```python
from build123d import *

# Parameters (mm, degrees)
EXTRUDE_1_DEPTH     = 5
FILLET_1_R          = 3
SKETCH_11_R         = 2
CUT_EXTRUDE_6_DEPTH = 88.5
SKETCH_12_R         = 2
CUT_EXTRUDE_7_DEPTH = 88.5


with BuildPart() as part:
    # 스케치1 → 보스-돌출1 (new body)
    with BuildSketch(Plane(origin=(0, 0, 0), x_dir=(1, 0, 0), z_dir=(0, 1, 0))):
        Polygon((-60, -30), (-30, -60), (-12.5, -60), (-12.5, -75), (12.5, -75), (12.5, -60), (30, -60), (60, -30), (60, -12.5), (75, -12.5), (75, 12.5), (60, 12.5), (60, 30), (30, 60), (12.5, 60), (12.5, 75), (-12.5, 75), (-12.5, 60), (-30, 60), (-60, 30), (-60, 12.5), (-75, 12.5), (-75, -12.5), (-60, -12.5), align=None)
    extrude(amount=EXTRUDE_1_DEPTH)

    # 필렛1
    fillet_1_edges = [part.edges().sort_by_distance(p)[0] for p in [
        (-12.5, 2.5, -75),
        (12.5, 2.5, -75),
        (75, 2.5, -12.5),
        (75, 2.5, 12.5),
        (12.5, 2.5, 75),
        (-12.5, 2.5, 75),
        (-75, 2.5, 12.5),
        (-75, 2.5, -12.5),
    ]]
    fillet(fillet_1_edges, radius=FILLET_1_R)

    # 스케치11 → 컷-돌출6 (cut, through all)
    with BuildSketch(Plane.XY.offset(12.5)):
        with Locations((-70, 2.5)):
            Circle(SKETCH_11_R)
        with Locations((70, 2.5)):
            Circle(SKETCH_11_R)
    extrude(amount=-CUT_EXTRUDE_6_DEPTH, mode=Mode.SUBTRACT)

    # 스케치12 → 컷-돌출7 (cut, through all)
    with BuildSketch(Plane.ZY.offset(12.5)):
        with Locations((-70, 2.5)):
            Circle(SKETCH_12_R)
        with Locations((70, 2.5)):
            Circle(SKETCH_12_R)
    extrude(amount=-CUT_EXTRUDE_7_DEPTH, mode=Mode.SUBTRACT)


solid = part.part
```
Geometry check sheet. Reference: the model listing, model coordinates, mm. A direction names the side the tool comes from. Coordinates: 2 decimals unless noted, no trailing zeros. Loops run counter-clockwise (first coordinate to the right, second up) from the corner with the lowest first, then second, coordinate; pieces in that order, holes last.
Item 1: Sectioned sample at D-D, the plane x = 50.5. Record the boundary of the cut face in (y, z), then the cut area to 3 significant figures.
Item 2: Sectioned sample at C-C, the plane z = 36.5. Record the boundary of the cut face in (x, y).
Item 3: Go/stop test with flat-tipped pins: pin 1 Ø2.5 at (y, z) = (2.5, 20.5) entering from -X; pin 2 Ø3 at (x, y) = (-28, 4) entering from -Z; pin 3 Ø2.5 at (y, z) = (1.5, 66) entering from -X. Record where each tip stops, or that it passes through.
Item 4: Sectioned sample at B-B, the plane z = -70. Record the boundary of the cut face in (x, y).
Item 5: Thickness scan on line 1 (Y direction, x = 70, z = -2); line 2 (Z direction, x = 2, y = 1.7); line 3 (Z direction, x = 61, y = 1.1). Record the ranges inside material, lowest first.
Item 6: Sectioned sample at A-A, the plane x = -70. Record the boundary of the cut face in (y, z).
Item 7: Release check for a two-part mould opening along Y. For faces 1 (the face through (71.908, 3.101, 0.175)), 2 (the face through (-1, 5, -1)), 3 (the face through (65, 2, -12.5)) record: released by +Y, released by -Y, zero draft, split by the parting line, or undercut.
Item 8: Access from +Z, -Z, +X, -X, +Y, -Y to the whole of each face (thin tool, end or side, straight path). Record for faces 4 (the face through (-65, 2, -12.5)), 5 (the face through (-12.5, 2, 65)), 6 (the face through (60, 2, -21)), 7 (the face through (65, 2, 12.5)).
Check result:
1. outline: (0, -39.5) - (5, -39.5) - (5, 39.5) - (0, 39.5) - close
1. area: 395 mm2
2. outline: (-53.5, 0) - (53.5, 0) - (53.5, 5) - (-53.5, 5) - close
3. pin 1: stops at x = -60
3. pin 2: stops at z = -60
3. pin 3: stops at x = -12.5
4. outline: (-12.5, 0) - (12.5, 0) - (12.5, 0.5) - (-12.5, 0.5) - close; (-12.5, 4.5) - (12.5, 4.5) - (12.5, 5) - (-12.5, 5) - close
5. line 1: y = 0 to 0.5, 4.5 to 5
5. line 2: z = -75 to -71.83, -68.17 to 68.17, 71.83 to 75
5. line 3: z = -12.5 to 12.5
6. outline: (0, -12.5) - (0.5, -12.5) - (0.5, 12.5) - (0, 12.5) - close; (4.5, -12.5) - (5, -12.5) - (5, 12.5) - (4.5, 12.5) - close
7. face 1: undercut
7. face 2: released by +Y
7. face 3: zero draft
8. face 4: -Z, -X, +Y, -Y
8. face 5: +Z, -X, +Y, -Y
8. face 6: -Z, +X, +Y, -Y
8. face 7: +Z, +X, +Y, -Y
